from build123d import *

# Parameters (mm, degrees)
F0_R     = 6
F0_R_2   = 4.25
F1_DEPTH = 5.5
F2_DEPTH = 2
F3_START = -4.5
F3_DEPTH = 1


with BuildPart() as f1:
    # F0 (on Top) → F1 (new body)
    with BuildSketch(Plane.XY):
        with BuildLine():
            ThreePointArc((5.5, -5.5), (15.7204938899, -4.6734816568), (25.6838378205, -2.2499706411))
            ThreePointArc((25.6838378205, -2.2499706411), (35.9990700802, 11.8329768619), (26, 26.1421356237))
            ThreePointArc((26, 26.1421356237), (-39, 21.6354367546), (-104, 26.1421356237))
            ThreePointArc((-104, 26.1421356237), (-113.4464485518, 7.9626587659), (-95.9436079124, -2.6853146853))
            ThreePointArc((-95.9436079124, -2.6853146853), (-59.6280544783, -0.4098034124), (-24.1395420925, -8.4449052422))
            ThreePointArc((-24.1395420925, -8.4449052422), (-14.2030574813, -15.5841269769), (-9.0771910213, -26.6939292452))
            Line((-9.0771910213, -26.6939292452), (-5.4164426416, -47.4550649772))
            ThreePointArc((-5.4164426416, -47.4550649772), (-3.5353318533, -50.7132444372), (0, -52))
            Line((0, -52), (3.5, -52))
            ThreePointArc((3.5, -52), (6.6819805153, -50.6819805153), (8, -47.5))
            Line((8, -47.5), (8, -46.5))
            Line((8, -46.5), (0, -46.5))
            Line((0, -46.5), (0, 0))
            Line((0, 0), (5.5, 0))
            Line((5.5, 0), (5.5, -5.5))
        make_face()
        with Locations((-99, 12)):
            Circle(F0_R, mode=Mode.SUBTRACT)
        with BuildLine():
            ThreePointArc((-69.8623954313, 5.5), (-77.9446739329, 5.2551191295), (-85.9973015672, 4.5213748947))
            ThreePointArc((-85.9973015672, 4.5213748947), (-84.0122690324, 11.3934355406), (-85.4354846008, 18.4034304857))
            ThreePointArc((-85.4354846008, 18.4034304857), (-39, 16.1354367546), (7.4354846008, 18.4034304857))
            ThreePointArc((7.4354846008, 18.4034304857), (6.0000953549, 11.9465150696), (7.4814941654, 5.5))
            Line((7.4814941654, 5.5), (-69.8623954313, 5.5))
        make_face(mode=Mode.SUBTRACT)
        with BuildLine():
            ThreePointArc((-5.4999999702, -19.4717688181), (-12.1799362134, -9.6798741804), (-22.1748882381, -3.3077722643))
            ThreePointArc((-22.1748882381, -3.3077722643), (-27.0245699268, -1.559616), (-31.9381287937, 0))
            Line((-31.9381287937, 0), (-5.4999999702, 0))
            Line((-5.4999999702, 0), (-5.4999999702, -19.4717688181))
        make_face(mode=Mode.SUBTRACT)
        with Locations((21, 12)):
            Circle(F0_R, mode=Mode.SUBTRACT)
        with Locations((21, 12)):
            Circle(F0_R)
        with Locations((21, 12)):
            Circle(F0_R_2, mode=Mode.SUBTRACT)
        with Locations((-99, 12)):
            Circle(F0_R)
        with Locations((-99, 12)):
            Circle(F0_R_2, mode=Mode.SUBTRACT)
    extrude(amount=-F1_DEPTH)

    # F0 (on Top) → F2 (join)
    with BuildSketch(Plane.XY):
        with Locations((21, 12)):
            Circle(F0_R)
        with Locations((21, 12)):
            Circle(F0_R_2, mode=Mode.SUBTRACT)
        with Locations((-99, 12)):
            Circle(F0_R)
        with Locations((-99, 12)):
            Circle(F0_R_2, mode=Mode.SUBTRACT)
    extrude(amount=F2_DEPTH)

    # F0 (on Top) → F3 (join)
    with BuildSketch(Plane.XY.offset(F3_START)):
        with BuildLine():
            ThreePointArc((-85.4354846008, 18.4034304857), (-84.0122690324, 11.3934355406), (-85.9973015672, 4.5213748947))
            ThreePointArc((-85.9973015672, 4.5213748947), (-77.9446739329, 5.2551191295), (-69.8623954313, 5.5))
            Line((-69.8623954313, 5.5), (7.4814941654, 5.5))
            ThreePointArc((7.4814941654, 5.5), (6.0000953549, 11.9465150696), (7.4354846008, 18.4034304857))
            ThreePointArc((7.4354846008, 18.4034304857), (-39, 16.1354367546), (-85.4354846008, 18.4034304857))
        make_face()
    extrude(amount=-F3_DEPTH)


solid = f1.part
Build history of the part. All positions in model axes, mm. A direction names the side the tool comes from. Coordinates: 2 decimals unless noted, no trailing zeros. Order: outer loops, then holes, each group sorted by start corner. A loop starts at its lowest first (then second) coordinate and runs counter-clockwise, first axis right, second up. Notation, with made-up numbers: (-28, 18.25) - (0, 18.25) arc R27 cw to (0, 35.25) - close; hole circle Ø5 at (-29, 40.25). An arc over 180 degrees is marked (long way). Write item = value, one per line. Start each with the question number.
1) 3-axis set-ups, long thin cutter, end or side, ignore diameter. For faces 4 (the face through (6.647, -50.717, -2.712)), 5 (the face through (-40, 12, -4.5)), 6 (the face through (3, 0, -3)): which of +Z, -Z, +X, -X, +Y, -Y reach the whole face in a straight line?
2) Flat gauge pins, fed straight in: pin 1 Ø4.5 at (x, z) = (3, -4) entering from +Y; pin 2 Ø1.5 at (x, y) = (-18.5, -15) entering from -Z; pin 3 Ø4.5 at (y, z) = (-14.5, -1.5) entering from -X; pin 4 Ø5 at (x, y) = (-63.5, 2.5) entering from +Z. Where does each tip first touch, or does it go through?
3) Two-plate mould, pull along X, no slides. Class faces 1 (the face through (-14.314, -15.451, -2.712)), 2 (the face through (36, 12, -3)), 3 (the face through (-77.832, 5.262, -2.218)): pulls with the +X half, pulls with the -X half, needs draft (parallel to the pull), parting line crosses it, or undercut.
4) Saw through at C-C on y = -15. Write the cut outline in (x, z), then the cut area to 3 significant figures.
5) Saw through at B-B on x = -26.5. Write the cut outline in (y, z), then the cut area to 3 significant figures.
6) Wall check: line 1 along Y through (x, z) = (-99, 1.5); line 2 along Z through (x, y) = (-12, -13.5); line 3 along Y through (x, z) = (23, 0.5). Give the ranges that are in metal, low to high. Write a range as from..to.
7) Saw through at D-D on z = -1.75. Write the cut outline in (x, y), then the cut area to 3 significant figures.
8) Saw through at A-A on y = 12. Write the cut outline in (x, z).
From the geometry:
q1.face_4 = +Z, -Z, +X, -Y
q1.face_5 = +Z
q1.face_6 = +Z, -Z
q2.pin_1 = 23.72
q2.pin_2 = through
q2.pin_3 = -17.56
q2.pin_4 = 0
q3.face_1 = pulls with the -X half
q3.face_2 = pulls with the +X half
q3.face_3 = undercut
q4.outline = (-14.7, -5.5) - (-7.84, -5.5) - (-7.84, 0) - (-14.7, 0) - close; (-5.5, -5.5) - (0, -5.5) - (0, 0) - (-5.5, 0) - close
q4.area = 68.0 mm^2
q5.outline = (-7.57, -5.5) - (-1.74, -5.5) - (-1.74, 0) - (-7.57, 0) - close; (0, -5.5) - (21.8, -5.5) - (21.8, 0) - (16.3, 0) - (16.3, -4.5) - (5.5, -4.5) - (5.5, 0) - (0, 0) - close
q5.area = 103 mm^2
q6.line_1 = 6..7.75, 16.25..18
q6.line_2 = -5.5..0
q6.line_3 = 6.34..8.25, 15.75..17.66
q7.outline = (-104, 26.14) arc R15 ccw to (-95.94, -2.69) arc R128 cw to (-24.14, -8.44) arc R24 cw to (-9.08, -26.69) - (-5.42, -47.46) arc R5.5 ccw to (0, -52) - (3.5, -52) arc R4.5 ccw to (8, -47.5) - (8, -46.5) - (0, -46.5) - (0, 0) - (5.5, 0) - (5.5, -5.5) arc R65 ccw to (25.68, -2.25) arc R15 ccw to (26, 26.14) arc R471 cw to start; hole circle Ø8.5 at (-99, 12); hole (-86, 4.52) arc R133.5 cw to (-69.86, 5.5) - (7.48, 5.5) arc R15 cw to (7.44, 18.4) arc R476.5 cw to (-85.44, 18.4) arc R15 cw to start; hole (-31.94, 0) arc R133.5 cw to (-22.17, -3.31) arc R29.5 cw to (-5.5, -19.47) - (-5.5, 0) - close; hole circle Ø8.5 at (21, 12)
q7.area = 3,030 mm^2
q8.outline = (-114, -5.5) - (-103.25, -5.5) - (-103.25, 2) - (-105, 2) - (-105, 0) - (-114, 0) - close; (-94.75, -5.5) - (16.75, -5.5) - (16.75, 2) - (15, 2) - (15, 0) - (6, 0) - (6, -4.5) - (-84, -4.5) - (-84, 0) - (-93, 0) - (-93, 2) - (-94.75, 2) - close; (25.25, -5.5) - (36, -5.5) - (36, 0) - (27, 0) - (27, 2) - (25.25, 2) - close
